Geometry: final body of the model. Coordinates: model frame, mm. Face numbers are marked on the shaded views. A direction names the side the tool comes from. Coordinates: 2 decimals unless noted, no trailing zeros. Write each loop counter-clockwise with the first axis right and the second up, starting at its lowest first coordinate (ties: lowest second). Pieces come first, ordered by that corner, then holes.
Autodesk Inventor part; units mm, degrees
ref_plane "Work Plane2" through (0, 0, 0.54) normal (0, 0, 1) x (1, 0, 0)
ref_plane "YZ Plane" through (0, 0, 0) normal (1, 0, 0) x (0, 1, 0)
ref_plane "XZ Plane" through (0, 0, 0) normal (0, 1, 0) x (-1, 0, 0)
sketch "Sketch1" plane through (0, 0, 0) normal (0, 0, 1) x (1, 0, 0)
  line L0 (0, 0) -> (0.4099, 0)
  line L1 (0, 0) -> (0, 0.6993)
  circle A0 centre (0, 0) radius 0.355
  line L2 (-1.725, 1.725) -> (1.725, 1.725) construction
  line L3 (1.725, 1.725) -> (1.725, -1.725) construction
  line L4 (1.725, -1.725) -> (-1.725, -1.725) construction
  line L5 (-1.725, -1.725) -> (-1.725, 1.725) construction
  line L6 (-1.725, 1.725) -> (-0.915, 1.725)
  line L7 (-0.915, 1.725) -> (-0.915, 0.915)
  line L8 (-0.915, 0.915) -> (-1.725, 0.915)
  line L9 (-1.725, 0.915) -> (-1.725, 1.725)
  line L10 (-1.725, -1.725) -> (-0.915, -1.725)
  line L11 (-0.915, -1.725) -> (-0.915, -0.915)
  line L12 (-0.915, -0.915) -> (-1.725, -0.915)
  line L13 (-1.725, -0.915) -> (-1.725, -1.725)
  line L14 (1.725, -1.725) -> (0.915, -1.725)
  line L15 (0.915, -1.725) -> (0.915, -0.915)
  line L16 (0.915, -0.915) -> (1.725, -0.915)
  line L17 (1.725, -0.915) -> (1.725, -1.725)
  line L18 (1.725, 1.725) -> (0.915, 1.725)
  line L19 (0.915, 1.725) -> (0.915, 0.915)
  line L20 (0.915, 0.915) -> (1.725, 0.915)
  line L21 (1.725, 0.915) -> (1.725, 1.725)
  dimension "d25" = 3.45
  dimension "d26" = 3.45
  dimension "d27" = 0.81
  dimension "d28" = 0.71
extrude "Extrusion1" add sketch "Sketch1" along normal blind 0.54
ref_plane "Work Plane2" through (0, 0, 0.54) normal (0, 0, 1) x (1, 0, 0)
sketch "Sketch2" plane through (0, 0, 0.54) normal (0, 0, 1) x (1, 0, 0)
  line L0 (-1.725, 1.725) -> (1.725, 1.725)
  line L1 (1.725, 1.725) -> (1.725, -1.725)
  line L2 (1.725, -1.725) -> (-1.725, -1.725)
  line L3 (-1.725, -1.725) -> (-1.725, 1.725)
  line L4 (0, 0) -> (0.4406, 0)
  line L5 (0, 0) -> (0, 0.4944)
extrude "Extrusion2" add sketch "Sketch2" along normal blind 1.03
sketch "Sketch3" plane through (0, 0, 1.57) normal (0, 0, 1) x (1, 0, 0)
  circle A0 centre (0, 0) radius 1.725
  circle A1 centre (0, 0) radius 1.5
  circle A2 centre (0, 0) radius 0.25
  dimension "d20" = 0.5
  dimension "d21" = 3.45
  dimension "d22" = 3
extrude "Extrusion3" add sketch "Sketch3" along normal blind 3.43
sketch "Sketch4" plane through (0, 0, 0) normal (0, 0, -1) x (-1, 0, 0)
  circle A0 centre (0, 0) radius 0.355
  circle A1 centre (0, 0) radius 0.355
  line L0 (-0.915, 0.915) -> (-1.515, 0.915)
  line L1 (-1.515, 0.915) -> (-1.515, 1.515)
  line L2 (-1.515, 1.515) -> (-0.915, 1.515)
  line L3 (-0.915, 1.515) -> (-0.915, 0.915)
  line L4 (0.915, 0.915) -> (1.515, 0.915)
  line L5 (1.515, 0.915) -> (1.515, 1.515)
  line L6 (1.515, 1.515) -> (0.915, 1.515)
  line L7 (0.915, 1.515) -> (0.915, 0.915)
  line L8 (0.915, -0.915) -> (1.515, -0.915)
  line L9 (1.515, -0.915) -> (1.515, -1.515)
  line L10 (1.515, -1.515) -> (0.915, -1.515)
  line L11 (0.915, -1.515) -> (0.915, -0.915)
  line L12 (-0.915, -0.915) -> (-1.515, -0.915)
  line L13 (-1.515, -0.915) -> (-1.515, -1.515)
  line L14 (-1.515, -1.515) -> (-0.915, -1.515)
  line L15 (-0.915, -1.515) -> (-0.915, -0.915)
  dimension "d29" = 0.6
extrude "Extrusion4" add sketch "Sketch4" along normal blind 1.7
properties part number "MMCX_thru" material "Brass, Soft Yellow"
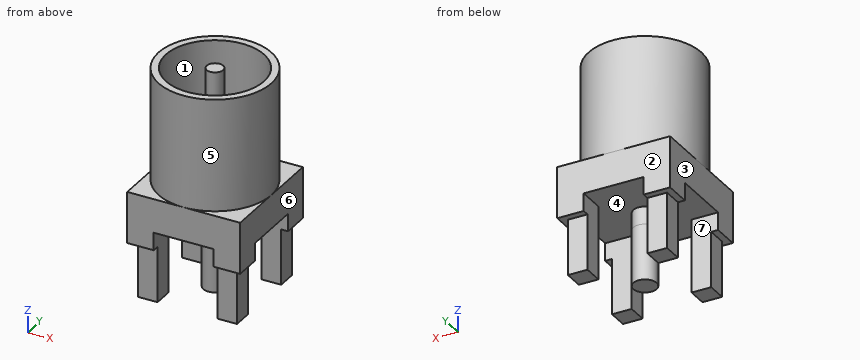
Item 1: Pin query (flat end, axial travel): pin 1 (1.5 mm diameter, centred on x = -1, z = 3, fed in from +Y); pin 2 (0.7 mm diameter, centred on x = -1, z = -0.5, fed in from +Y) (3 decimals); pin 3 (0.5 mm diameter, centred on x = -1, y = 0.5, fed in from +Z). Return the tip coordinate at first contact, or that it passes through.
Derived:
pin 1: stops at y = 1.71
pin 2: stops at y = 1.515
pin 3: stops at z = 1.57
Item 2: Section A-A, the plane z = 1.75. Output: boundary loops of the cut face in (x, y) (3 decimals), plus the area to 3 significant figures.
Derived:
outline: circle Ø3.45 at (0, 0); circle Ø0.5 at (0, 0); hole circle Ø3 at (0, 0)
area: 2.48 mm2
Item 3: Pull-direction query (X, two-part tool) for the marked faces 1, 2, 3 and 4; classes: released by +X, released by -X, zero draft, split by the parting line, or undercut.
Derived:
face 1: undercut
face 2: zero draft
face 3: released by -X
face 4: undercut
Item 4: Section B-B, the plane x = 0.5. Output: boundary loops of the cut face in (y, z) (3 decimals).
Derived:
outline: (-1.725, 0.54) - (1.725, 0.54) - (1.725, 1.57) - (1.651, 1.57) - (1.651, 5) - (1.414, 5) - (1.414, 1.57) - (-1.414, 1.57) - (-1.414, 5) - (-1.651, 5) - (-1.651, 1.57) - (-1.725, 1.57) - close
Item 5: Section C-C, the plane y = -1.3. Output: boundary loops of the cut face in (x, z) (3 decimals), plus the area to 3 significant figures.
Derived:
outline: (-1.725, 0) - (-1.515, 0) - (-1.515, -1.7) - (-0.915, -1.7) - (-0.915, 0.54) - (0.915, 0.54) - (0.915, -1.7) - (1.515, -1.7) - (1.515, 0) - (1.725, 0) - (1.725, 1.57) - (1.134, 1.57) - (1.134, 5) - (0.748, 5) - (0.748, 1.57) - (-0.748, 1.57) - (-0.748, 5) - (-1.134, 5) - (-1.134, 1.57) - (-1.725, 1.57) - close
area: 9.11 mm2
Item 6: Section D-D, the plane y = 0.75. Output: boundary loops of the cut face in (x, z) (3 decimals).
Derived:
outline: (-1.725, 0.54) - (1.725, 0.54) - (1.725, 1.57) - (1.553, 1.57) - (1.553, 5) - (1.299, 5) - (1.299, 1.57) - (-1.299, 1.57) - (-1.299, 5) - (-1.553, 5) - (-1.553, 1.57) - (-1.725, 1.57) - close
Item 7: Set-up query: the marked faces 5, 6 and 7. Return all of +Z, -Z, +X, -X, +Y, -Y with unobstructed straight access to the full face (end or side cutting, diameter ignored); none if empty.
Derived:
face 5: +Z
face 6: +Z, -Z, +X, +Y, -Y
face 7: -Z, +X, -X
Item 8: Material intervals for probe 1 along Y at (x, z) = (0, 3.45) (3 decimals); probe 2 along Z at (x, y) = (-1, 0.05); probe 3 along X at (y, z) = (-0.65, 2.75), sorted ascending.
Derived:
probe 1: y = -1.725 to -1.5, -0.25 to 0.25, 1.5 to 1.725
probe 2: z = 0.54 to 1.57
probe 3: x = -1.6 to -1.35, 1.35 to 1.6
